```python
from build123d import *

# Parameters (mm, degrees)
SKETCH_R        = 3.6
SKETCH_R_2      = 1.6
SKETCH_W        = 6.5
SKETCH_H        = 3
SKETCH_W_2      = 11.5
PAD_DEPTH       = 9
POCKET_DEPTH    = 2.6
POCKET001_DEPTH = 7
SKETCH003_W     = 25.7
SKETCH003_H     = 13
POCKET002_DEPTH = 3
SKETCH004_R     = 1.8
POCKET003_DEPTH = 2
SKETCH005_W     = 9
SKETCH005_H     = 2.6
POCKET004_DEPTH = 9.001
CHAMFER_SIZE    = 5
FILLET_R        = 1
FILLET001_R     = 0.99
FILLET002_R     = 0.5


with BuildPart() as part:
    # Sketch → Pad (new body)
    with BuildSketch(Plane.XY):
        with BuildLine():
            Line((15.5, -31.15), (15.5, -6.75))
            Line((15.5, -6.75), (11.5, -6.75))
            Line((11.5, -6.75), (11.5, 6.75))
            Line((11.5, 6.75), (15.5, 6.75))
            Line((15.5, 6.75), (15.5, 11.85))
            Line((15.5, 11.85), (-15.5, 11.85))
            Line((-15.5, 11.85), (-15.5, -25.7))
            ThreePointArc((-15.5, -25.7), (-14.679899, -27.679899), (-12.7, -28.5))
            Line((-11.7, -28.5), (-12.7, -28.5))
            Line((-11.7, -29.15), (-11.7, -28.5))
            ThreePointArc((-11.7, -29.15), (-11.114214, -30.564214), (-9.7, -31.15))
            Line((-9.7, -31.15), (15.5, -31.15))
        make_face()
        Circle(SKETCH_R, mode=Mode.SUBTRACT)
        with Locations((-11, -12.5)):
            Circle(SKETCH_R_2, mode=Mode.SUBTRACT)
        with Locations((11, -12.5)):
            Circle(SKETCH_R_2, mode=Mode.SUBTRACT)
        with Locations((-6, 8.5)):
            Circle(SKETCH_R_2, mode=Mode.SUBTRACT)
        with Locations((8, 8.5)):
            Circle(SKETCH_R_2, mode=Mode.SUBTRACT)
        with Locations((-8.91, -25.81)):
            Rectangle(SKETCH_W, SKETCH_H, mode=Mode.SUBTRACT)
        with Locations((6.35, -25.81)):
            Rectangle(SKETCH_W_2, SKETCH_H, mode=Mode.SUBTRACT)
    extrude(amount=PAD_DEPTH)

    # Sketch001 (on Face28 of Pad) → Pocket (cut)
    with BuildSketch(Plane.XY.offset(9)):
        Polygon((-8.1, -14.174316), (-8.1, -10.825684), (-11, -9.151368), (-13.9, -10.825684), (-13.9, -14.174316), (-11, -15.848632), align=None)
        Polygon((13.9, -14.174316), (13.9, -10.825684), (11, -9.151368), (8.1, -10.825684), (8.1, -14.174316), (11, -15.848632), align=None)
    extrude(amount=-POCKET_DEPTH, mode=Mode.SUBTRACT)

    # Sketch002 → Pocket001 (cut)
    with BuildSketch(Plane(origin=(0, 0, 0), x_dir=(1, 0, 0), z_dir=(0, 0, -1))):
        Polygon((8.25, -4), (6.25, -4), (6.25, -6.25), (-6.25, -6.25), (-6.25, -4), (-8.25, -4), (-8.25, 4), (-6.25, 4), (-6.25, 6.25), (6.25, 6.25), (6.25, 4), (8.25, 4), align=None)
    extrude(amount=-POCKET001_DEPTH, mode=Mode.SUBTRACT)

    # Sketch003 → Pocket002 (cut)
    with BuildSketch(Plane(origin=(0, 0, 0), x_dir=(1, 0, 0), z_dir=(0, 0, -1))):
        with Locations((0, 22)):
            Rectangle(SKETCH003_W, SKETCH003_H)
    extrude(amount=-POCKET002_DEPTH, mode=Mode.SUBTRACT)

    # Sketch004 (on Face56 of Pocket002) → Pocket003 (cut)
    with BuildSketch(Plane(origin=(0, 0, 3), x_dir=(1, 0, 0), z_dir=(0, 0, -1))):
        with Locations((0, 22)):
            Circle(SKETCH004_R)
        with BuildLine():
            Line((1.5, 15.5), (12.85, 15.5))
            Line((12.85, 15.5), (12.85, 20.5))
            Line((12.85, 20.5), (3.5, 20.5))
            ThreePointArc((3.5, 20.5), (2.085786, 19.914214), (1.5, 18.5))
            Line((1.5, 18.5), (1.5, 15.5))
        make_face()
        with BuildLine():
            Line((-1.5, 15.5), (-12.85, 15.5))
            Line((-12.85, 15.5), (-12.85, 20.5))
            Line((-12.85, 20.5), (-3.5, 20.5))
            ThreePointArc((-1.5, 18.5), (-2.085786, 19.914214), (-3.5, 20.5))
            Line((-1.5, 18.5), (-1.5, 15.5))
        make_face()
        with BuildLine():
            Line((12.85, 23.5), (3.5, 23.5))
            ThreePointArc((1.5, 25.5), (2.085786, 24.085786), (3.5, 23.5))
            Line((1.5, 25.5), (1.5, 28.5))
            Line((1.5, 28.5), (12.85, 28.5))
            Line((12.85, 28.5), (12.85, 23.5))
        make_face()
        with BuildLine():
            Line((-12.85, 23.5), (-3.5, 23.5))
            ThreePointArc((-3.5, 23.5), (-2.085786, 24.085786), (-1.5, 25.5))
            Line((-1.5, 25.5), (-1.5, 28.5))
            Line((-1.5, 28.5), (-12.85, 28.5))
            Line((-12.85, 28.5), (-12.85, 23.5))
        make_face()
    extrude(amount=-POCKET003_DEPTH, mode=Mode.SUBTRACT)

    # Sketch005 (on Face5 of Pocket003) → Pocket004 (cut, through all)
    with BuildSketch(Plane.XY.offset(9)):
        with Locations((2.54, -13.11)):
            Rectangle(SKETCH005_W, SKETCH005_H)
    extrude(amount=-POCKET004_DEPTH, mode=Mode.SUBTRACT)

    # Chamfer
    chamfer_edges = [part.edges().sort_by_distance(p)[0] for p in [
        (-15.5, 11.85, 4.5),
    ]]
    chamfer(chamfer_edges, length=CHAMFER_SIZE)

    # Fillet
    fillet_edges = [part.edges().sort_by_distance(p)[0] for p in [
        (-10.5, 11.85, 4.5),
        (-15.5, 6.85, 4.5),
        (15.5, 11.85, 4.5),
        (15.5, -6.75, 4.5),
        (15.5, 6.75, 4.5),
        (15.5, -31.15, 4.5),
        (-12.16, -24.31, 7),
        (-5.66, -24.31, 7),
        (-5.66, -27.31, 7),
        (12.1, -27.31, 7),
        (12.1, -24.31, 7),
        (0.6, -24.31, 6),
        (0.6, -27.31, 6),
        (-12.16, -27.31, 7),
        (-1.96, -11.81, 4.5),
        (7.04, -11.81, 4.5),
        (7.04, -14.41, 4.5),
        (-1.96, -14.41, 4.5),
    ]]
    fillet(fillet_edges, radius=FILLET_R)

    # Fillet001
    fillet001_edges = [part.edges().sort_by_distance(p)[0] for p in [
        (-6.25, -4, 3.5),
        (-8.25, -4, 3.5),
        (-6.25, -6.25, 3.5),
        (6.25, -6.25, 3.5),
        (6.25, -4, 3.5),
        (8.25, -4, 3.5),
        (-8.25, 4, 3.5),
        (-6.25, 4, 3.5),
        (-6.25, 6.25, 3.5),
        (8.25, 4, 3.5),
        (6.25, 4, 3.5),
        (6.25, 6.25, 3.5),
    ]]
    fillet(fillet001_edges, radius=FILLET001_R)

    # Fillet002
    fillet002_edges = [part.edges().sort_by_distance(p)[0] for p in [
        (11.5, 6.75, 4.5),
        (11.5, -6.75, 4.5),
        (-12.85, -15.5, 4),
        (-12.85, -15.5, 1.5),
        (-12.85, -20.5, 4),
        (-12.85, -23.5, 4),
        (12.85, -20.5, 4),
        (12.85, -15.5, 4),
        (12.85, -15.5, 1.5),
        (12.85, -28.5, 4),
        (12.85, -28.5, 1.5),
        (12.85, -23.5, 4),
        (1.5, -27.304987, 4),
        (-11.7, -28.5, 7),
    ]]
    fillet(fillet002_edges, radius=FILLET002_R)


solid = part.part
```
The listing builds one solid part. Answer for the finished solid, in the listing's coordinates (mm). A direction names the side the tool comes from. Give positions to 0.01 mm unless a question says otherwise; leave off trailing zeros. Order: outer loops, then holes, each group sorted by start corner. A loop starts at its lowest first (then second) coordinate and runs counter-clockwise, first axis right, second up. Notation, with made-up numbers: (86.5, -26.75) -> (112.5, -26.75) arc R22 ccw to (112.5, -4.75) -> close; hole circle Ø7 at (6, 52.25). An arc over 180 degrees is marked (long way). Answer as CSV lines item,"result". Start each with the question number.
Q1. A cutting plane is placed at B-B (y = 8.5). Determine the outline of the cut face in (x, z).
Q2. A cutting plane is placed at C-C (x = 0). Determine the outline of the cut face in (y, z), then the cut area to 4 significant figures.
Q3. A cutting plane is placed at D-D (z = 2). Count the separate pieces of the cut face and the enclosed holes in it, then the cut area to 3 significant figures.
Q4. Given pin 1 (1.5 mm diameter, centred on x = 0, y = -27, fed in from -Z); pin 2 (1.8 mm diameter, centred on y = -0.5, z = 3.5, fed in from +X), each flat-ended and moving along its own axis, determine where each tip first touches the part or whether it passes through.
Q5. Which of the six approach directions +Z, -Z, +X, -X, +Y, -Y give full straight-line access (tool end or side, diameter ignored) to faces 1 (the cylindrical face through (6.739, -14.125, 4.437)), 2 (the flat face through (1.5, -28, 4)), 3 (the flat face through (-9.53, -10, 7.72)), 4 (the flat face through (11.5, 0, 4))?
Q6. A cutting plane is placed at A-A (y = 0). Determine the outline of the cut face in (x, z).
Q7. Determine the mould class of faces 5 (the flat face through (-13.03, 9.32, 4.44)), 6 (the flat face through (2, -31.15, 4)), 7 (the cylindrical face through (6.55, -4.28, 3.55)), 8 (the flat face through (15.5, -19, 4)) for opening direction Y: pulls with the +Y half, pulls with the -Y half, needs draft (parallel to the pull), parting line crosses it, or undercut.
Q8. Find the intervals of material crossed by L1, parallel to Y at x = 6, z = 7.5; L2, parallel to Y at x = 0, z = 8.15; L3, parallel to X at y = 0, z = 7.9, in increasing order.
Results found:
1,outline,"(-13.85, 0) -> (-7.6, 0) -> (-7.6, 9) -> (-13.85, 9) -> close; (-4.4, 0) -> (6.4, 0) -> (6.4, 9) -> (-4.4, 9) -> close; (9.6, 0) -> (15.5, 0) -> (15.5, 9) -> (9.6, 9) -> close"
2,outline,"(-31.15, 0) -> (-28.5, 0) -> (-28.5, 3) -> (-23.8, 3) -> (-23.8, 5) -> (-20.2, 5) -> (-20.2, 3) -> (-15.5, 3) -> (-15.5, 0) -> (-14.41, 0) -> (-14.41, 9) -> (-31.15, 9) -> close; (-11.81, 0) -> (-6.25, 0) -> (-6.25, 7) -> (-3.6, 7) -> (-3.6, 9) -> (-11.81, 9) -> close; (3.6, 7) -> (6.25, 7) -> (6.25, 0) -> (11.85, 0) -> (11.85, 9) -> (3.6, 9) -> close"
2,area,"215.5 mm2"
3,separate pieces,"1"
3,enclosed holes,"6"
3,area,"677 mm2"
4,pin 1,"z = 3"
4,pin 2,"x = 11.5"
5,face 1,"+Z, -Z"
5,face 2,"-Z"
5,face 3,"+Z"
5,face 4,"+Z, -Z, +X"
6,outline,"(-15.5, 0) -> (-8.25, 0) -> (-8.25, 7) -> (-3.6, 7) -> (-3.6, 9) -> (-15.5, 9) -> close; (3.6, 7) -> (8.25, 7) -> (8.25, 0) -> (11.5, 0) -> (11.5, 9) -> (3.6, 9) -> close"
7,face 5,"pulls with the +Y half"
7,face 6,"pulls with the -Y half"
7,face 7,"undercut"
7,face 8,"needs draft"
8,L1,"-31.15 to -27.31, -24.31 to -14.41, -11.81 to 11.85"
8,L2,"-31.15 to -14.41, -11.81 to -3.6, 3.6 to 11.85"
8,L3,"-15.5 to -3.6, 3.6 to 11.5"
